Part model, mm, in its own coordinate system. Face numbers are marked on the shaded views. Round coordinates to 2 decimals unless told otherwise and drop trailing zeros. Loops run counter-clockwise (first coordinate to the right, second up) from the corner with the lowest first, then second, coordinate; pieces in that order, holes last.
1) Band-saw the part on A-A, the plane x = -49. Write the cut outline in (y, z), then the cut area to 3 significant figures.
2) Drop flat-ended pins along their axis: P1, Ø0.5, axis at x = 59, y = 0.5, coming from the +Z side; P2, Ø5, axis at x = 72.5, z = 68, coming from the -Y side; P3, Ø1, axis at y = 10.5, z = -46.5, coming from the -X side; P4, Ø2.5, axis at x = -72.5, z = -68, coming from the +Y side. Give the stop position or say it passes through.
3) Probe line 1 (X direction, y = 5.3, z = -68); line 2 (Z direction, x = 2.5, y = 6.25); line 3 (Z direction, x = 72.5, y = 4.6). List the from-to ranges inside material, lowest first.
4) Band-saw the part on B-B, the plane z = 12. Write the cut outline in (x, y).
5) Mould opens along X. For the marked faces 1, 2 and 3 say: +X half, -X half, draft (parallel to the pull), parting line (faces both ways), or undercut.
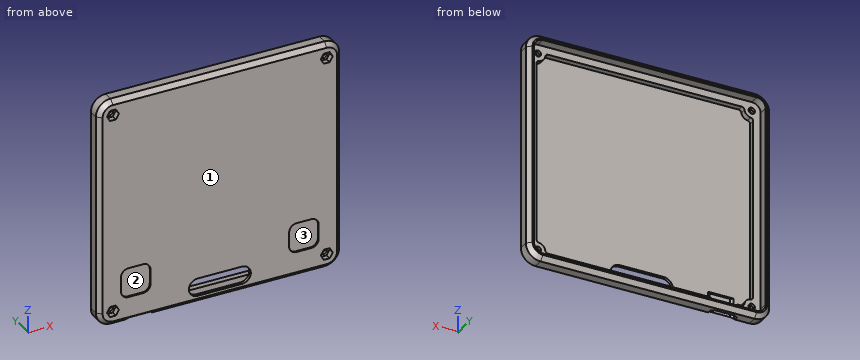
from build123d import *

# Parameters (mm, degrees)
BOSS_EXTRUDE2_DEPTH      = 2
BOSS_EXTRUDE3_DEPTH      = 4
BOSS_EXTRUDE3_DEPTH_BACK = 2
SKETCH3_R                = 2.15
BOSS_EXTRUDE4_DEPTH      = 6.38
CUT_EXTRUDE1_DEPTH       = 15
FILLET1_R                = 2
CUT_EXTRUDE3_DEPTH       = 115.008747033
CUT_EXTRUDE3_DEPTH_BACK  = 115.008747033
SKETCH11_R               = 2.15
CUT_EXTRUDE2_DEPTH       = 4
CHAMFER1_SIZE            = 3
SKETCH13_W               = 18
SKETCH13_H               = 5
CUT_EXTRUDE5_DEPTH       = 1
CUT_EXTRUDE6_DEPTH       = 1
CUT_EXTRUDE7_DEPTH       = 2


with BuildPart() as part:
    # Sketch2 → Boss-Extrude2 (new body)
    with BuildSketch(Plane(origin=(0, 0, 0), x_dir=(1, 0, 0), z_dir=(0, 1, 0))):
        with BuildLine():
            Line((-72.5, 74), (72.5, 74))
            ThreePointArc((72.5, 74), (76.742640687, 72.242640687), (78.5, 68))
            Line((78.5, 68), (78.5, -68))
            ThreePointArc((78.5, -68), (76.742640687, -72.242640687), (72.5, -74))
            Line((72.5, -74), (-72.5, -74))
            ThreePointArc((-72.5, -74), (-76.742640687, -72.242640687), (-78.5, -68))
            Line((-78.5, -68), (-78.5, 68))
            ThreePointArc((-78.5, 68), (-76.742640687, 72.242640687), (-72.5, 74))
        make_face()
    extrude(amount=BOSS_EXTRUDE2_DEPTH)

    # Sketch3 → Boss-Extrude3 (add, two sides: drawn at the far end of the back side and taken through both)
    with BuildSketch(Plane(origin=(0, 2, 0), x_dir=(1, 0, 0), z_dir=(0, 1, 0)).offset(-BOSS_EXTRUDE3_DEPTH_BACK)):
        with BuildLine():
            Line((-82.5, 68), (-82.5, -68))
            ThreePointArc((-82.5, -68), (-79.571067812, -75.071067812), (-72.5, -78))
            Line((-72.5, -78), (72.5, -78))
            ThreePointArc((72.5, -78), (79.571067812, -75.071067812), (82.5, -68))
            Line((82.5, -68), (82.5, 68))
            ThreePointArc((82.5, 68), (79.571067812, 75.071067812), (72.5, 78))
            Line((72.5, 78), (-72.5, 78))
            ThreePointArc((-72.5, 78), (-79.571067812, 75.071067812), (-82.5, 68))
        make_face()
        with Locations(Location((-72.5, -68, 0), (0, 0, 270))):
            Circle(SKETCH3_R, mode=Mode.SUBTRACT)
        with Locations(Location((72.5, -68, 0), (0, 0, 270))):
            Circle(SKETCH3_R, mode=Mode.SUBTRACT)
        with Locations(Location((72.5, 68, 0), (0, 0, 270))):
            Circle(SKETCH3_R, mode=Mode.SUBTRACT)
        with Locations(Location((-72.5, 68, 0), (0, 0, 270))):
            Circle(SKETCH3_R, mode=Mode.SUBTRACT)
        with BuildLine():
            Line((-73.5, 63), (-73.5, -63))
            Line((-73.5, -63), (-72.5, -63))
            ThreePointArc((-72.5, -63), (-68.964466094, -64.464466094), (-67.5, -68))
            Line((-67.5, -68), (-67.5, -69))
            Line((-67.5, -69), (67.5, -69))
            Line((67.5, -69), (67.5, -68))
            ThreePointArc((67.5, -68), (68.964466094, -64.464466094), (72.5, -63))
            Line((72.5, -63), (73.5, -63))
            Line((73.5, -63), (73.5, 63))
            Line((73.5, 63), (72.5, 63))
            ThreePointArc((72.5, 63), (68.964466094, 64.464466094), (67.5, 68))
            Line((67.5, 68), (67.5, 69))
            Line((67.5, 69), (-67.5, 69))
            Line((-67.5, 69), (-67.5, 68))
            ThreePointArc((-67.5, 68), (-68.964466094, 64.464466094), (-72.5, 63))
            Line((-72.5, 63), (-73.5, 63))
        make_face(mode=Mode.SUBTRACT)
    extrude(amount=BOSS_EXTRUDE3_DEPTH + BOSS_EXTRUDE3_DEPTH_BACK)

    # Sketch8 → Boss-Extrude4 (add)
    with BuildSketch(Plane(origin=(0, 6, 0), x_dir=(1, 0, 0), z_dir=(0, 1, 0))):
        with BuildLine():
            ThreePointArc((82.5, 68), (79.571067812, 75.071067812), (72.5, 78))
            Line((72.5, 78), (-72.5, 78))
            ThreePointArc((-72.5, 78), (-79.571067812, 75.071067812), (-82.5, 68))
            Line((-82.5, 68), (-82.5, -68))
            ThreePointArc((-82.5, -68), (-79.571067812, -75.071067812), (-72.5, -78))
            Line((-72.5, -78), (72.5, -78))
            ThreePointArc((72.5, -78), (79.571067812, -75.071067812), (82.5, -68))
            Line((82.5, -68), (82.5, 68))
        make_face()
        with BuildLine():
            ThreePointArc((72.5, -74), (76.742640687, -72.242640687), (78.5, -68))
            Line((78.5, -68), (78.5, 68))
            ThreePointArc((78.5, 68), (76.742640687, 72.242640687), (72.5, 74))
            Line((72.5, 74), (-72.5, 74))
            ThreePointArc((-72.5, 74), (-76.742640687, 72.242640687), (-78.5, 68))
            Line((-78.5, 68), (-78.5, -68))
            ThreePointArc((-78.5, -68), (-76.742640687, -72.242640687), (-72.5, -74))
            Line((-72.5, -74), (72.5, -74))
        make_face(mode=Mode.SUBTRACT)
    extrude(amount=BOSS_EXTRUDE4_DEPTH)

    # Sketch9 → Cut-Extrude1 (cut)
    with BuildSketch(Plane(origin=(0, 0, -78), x_dir=(-1, 0, 0), z_dir=(0, 0, -1))):
        Polygon((60.62, 7.11), (46.62, 7.11), (44.62, 5.51), (44.62, 2.19), (46.62, 0.59), (60.62, 0.59), (62.62, 2.19), (62.62, 5.51), align=None)
    extrude(amount=-CUT_EXTRUDE1_DEPTH, mode=Mode.SUBTRACT)

    # Fillet1
    fillet1_edges = [part.edges().sort_by_distance(p)[0] for p in [
        (-67.5, 4, -69),
        (-73.5, 4, -63),
        (-73.5, 4, 63),
        (-67.5, 4, 69),
        (73.5, 4, 63),
        (67.5, 4, 69),
        (67.5, 4, -69),
        (73.5, 4, -63),
    ]]
    fillet(fillet1_edges, radius=FILLET1_R)

    # Sketch11 → Cut-Extrude3 (cut, two sides: drawn at the far end of the back side and taken through both)
    with BuildSketch(Plane(origin=(0, 2, 0), x_dir=(1, 0, 0), z_dir=(0, 1, 0)).offset(-CUT_EXTRUDE3_DEPTH_BACK)):
        with Locations(Location((-72.5, -68, 0), (0, 0, 270))):
            Circle(SKETCH11_R)
        with Locations(Location((72.5, -68, 0), (0, 0, 270))):
            Circle(SKETCH11_R)
        with Locations(Location((72.5, 68, 0), (0, 0, 270))):
            Circle(SKETCH11_R)
        with Locations(Location((-72.5, 68, 0), (0, 0, 270))):
            Circle(SKETCH11_R)
    extrude(amount=CUT_EXTRUDE3_DEPTH + CUT_EXTRUDE3_DEPTH_BACK, mode=Mode.SUBTRACT)

    # Sketch10 → Cut-Extrude2 (cut)
    with BuildSketch(Plane.XZ):
        Polygon((-74.520725942, 64.5), (-70.479274058, 64.5), (-68.458548116, 68), (-70.479274058, 71.5), (-74.520725942, 71.5), (-76.541451884, 68), align=None)
        Polygon((76.541451884, 68), (74.520725942, 64.5), (70.479274058, 64.5), (68.458548116, 68), (70.479274058, 71.5), (74.520725942, 71.5), align=None)
        Polygon((-70.479274058, -64.5), (-68.458548116, -68), (-70.479274058, -71.5), (-74.520725942, -71.5), (-76.541451884, -68), (-74.520725942, -64.5), align=None)
        Polygon((76.541451884, -68), (74.520725942, -64.5), (70.479274058, -64.5), (68.458548116, -68), (70.479274058, -71.5), (74.520725942, -71.5), align=None)
    extrude(amount=-CUT_EXTRUDE2_DEPTH, mode=Mode.SUBTRACT)

    # Chamfer1
    # the kernel refuses this chamfer: 3 mm, written as the material it takes off along each edge
    with BuildSketch(Plane(origin=(-72.5, 12.38, 68), x_dir=(-1, 0, 0), z_dir=(0, 0, -1))) as chamfer1_piece_1:
        Polygon((10 - CHAMFER1_SIZE, 0), (10, -CHAMFER1_SIZE), (10, 0), align=None)
    revolve(axis=Axis((-72.5, 12.38, 68), (0, 1, 0)), revolution_arc=90, mode=Mode.SUBTRACT)
    with BuildSketch(Plane(origin=(-72.5, 12.38, 78), x_dir=(0, 0.02749587661058619, -0.9996219169112968), z_dir=(1, 0, 0)), Plane(origin=(72.5, 0, -78), x_dir=(0, 0.9996219169112968, -0.027495876610586778), z_dir=(-1, 0, 0))) as chamfer1_piece_2:
        Polygon((CHAMFER1_SIZE * 0.999621916911, -CHAMFER1_SIZE * 0.0274958766106), (-CHAMFER1_SIZE * 0.0274958766106, -CHAMFER1_SIZE * 0.999621916911), (0, 0), align=None)
    extrude(amount=145, mode=Mode.SUBTRACT)
    with BuildSketch(Plane(origin=(72.5, 12.38, 68), x_dir=(0, 0, 1), z_dir=(-1, 0, 0))) as chamfer1_piece_3:
        Polygon((10 - CHAMFER1_SIZE, 0), (10, -CHAMFER1_SIZE), (10, 0), align=None)
    revolve(axis=Axis((72.5, 12.38, 68), (0, 1, 0)), revolution_arc=90, mode=Mode.SUBTRACT)
    with BuildSketch(Plane(origin=(82.5, 12.38, 68), x_dir=(-0.9996219169112968, 0.02749587661058619, 0), z_dir=(0, 0, -1)), Plane(origin=(-82.5, 12.38, -68), x_dir=(0.9996219169112968, 0.02749587661058619, 0), z_dir=(0, 0, 1))) as chamfer1_piece_4:
        Polygon((CHAMFER1_SIZE * 0.999621916911, -CHAMFER1_SIZE * 0.0274958766106), (-CHAMFER1_SIZE * 0.0274958766106, -CHAMFER1_SIZE * 0.999621916911), (0, 0), align=None)
    extrude(amount=136, mode=Mode.SUBTRACT)
    with BuildSketch(Plane(origin=(72.5, 12.38, -68), x_dir=(1, 0, 0), z_dir=(0, 0, 1))) as chamfer1_piece_5:
        Polygon((10 - CHAMFER1_SIZE, 0), (10, -CHAMFER1_SIZE), (10, 0), align=None)
    revolve(axis=Axis((72.5, 12.38, -68), (0, 1, 0)), revolution_arc=90, mode=Mode.SUBTRACT)
    with BuildSketch(Plane(origin=(72.5, 12.38, -78), x_dir=(0, -0.9996219169112968, -0.02749587661058678), z_dir=(-1, 0, 0)), Plane(origin=(-72.5, 0, 78), x_dir=(0, -0.02749587661058636, -0.9996219169112968), z_dir=(1, 0, 0))) as chamfer1_piece_6:
        Polygon((CHAMFER1_SIZE * 0.999621916911, CHAMFER1_SIZE * 0.0274958766106), (-CHAMFER1_SIZE * 0.0274958766106, CHAMFER1_SIZE * 0.999621916911), (0, 0), align=None)
    extrude(amount=145, mode=Mode.SUBTRACT)
    with BuildSketch(Plane(origin=(-72.5, 12.38, -68), x_dir=(0, 0, -1), z_dir=(1, 0, 0))) as chamfer1_piece_7:
        Polygon((10 - CHAMFER1_SIZE, 0), (10, -CHAMFER1_SIZE), (10, 0), align=None)
    revolve(axis=Axis((-72.5, 12.38, -68), (0, 1, 0)), revolution_arc=90, mode=Mode.SUBTRACT)
    with BuildSketch(Plane(origin=(-72.5, 0, -68), x_dir=(0, 0, -1), z_dir=(1, 0, 0))) as chamfer1_piece_8:
        Polygon((10 - CHAMFER1_SIZE, 0), (10, CHAMFER1_SIZE), (10, 0), align=None)
    revolve(axis=Axis((-72.5, 0, -68), (0, 1, 0)), revolution_arc=90, mode=Mode.SUBTRACT)
    with BuildSketch(Plane(origin=(-82.5, 0, -68), x_dir=(0.9996219169112968, -0.02749587661058636, 0), z_dir=(0, 0, 1)), Plane(origin=(82.5, 0, 68), x_dir=(-0.9996219169112968, -0.02749587661058636, 0), z_dir=(0, 0, -1))) as chamfer1_piece_9:
        Polygon((CHAMFER1_SIZE * 0.999621916911, CHAMFER1_SIZE * 0.0274958766106), (-CHAMFER1_SIZE * 0.0274958766106, CHAMFER1_SIZE * 0.999621916911), (0, 0), align=None)
    extrude(amount=136, mode=Mode.SUBTRACT)
    with BuildSketch(Plane(origin=(-72.5, 0, 68), x_dir=(-1, 0, 0), z_dir=(0, 0, -1))) as chamfer1_piece_10:
        Polygon((10 - CHAMFER1_SIZE, 0), (10, CHAMFER1_SIZE), (10, 0), align=None)
    revolve(axis=Axis((-72.5, 0, 68), (0, 1, 0)), revolution_arc=90, mode=Mode.SUBTRACT)
    with BuildSketch(Plane(origin=(72.5, 0, 68), x_dir=(0, 0, 1), z_dir=(-1, 0, 0))) as chamfer1_piece_11:
        Polygon((10 - CHAMFER1_SIZE, 0), (10, CHAMFER1_SIZE), (10, 0), align=None)
    revolve(axis=Axis((72.5, 0, 68), (0, 1, 0)), revolution_arc=90, mode=Mode.SUBTRACT)
    with BuildSketch(Plane(origin=(72.5, 0, -68), x_dir=(1, 0, 0), z_dir=(0, 0, 1))) as chamfer1_piece_12:
        Polygon((10, CHAMFER1_SIZE), (10 - CHAMFER1_SIZE, 0), (10, 0), align=None)
    revolve(axis=Axis((72.5, 0, -68), (0, 1, 0)), revolution_arc=90, mode=Mode.SUBTRACT)

    # Sketch13 → Cut-Extrude5 (cut)
    with BuildSketch(Plane(origin=(0, 6, 0), x_dir=(1, 0, 0), z_dir=(0, 1, 0))):
        with Locations((-53.62, 71.5)):
            Rectangle(SKETCH13_W, SKETCH13_H)
    extrude(amount=-CUT_EXTRUDE5_DEPTH, mode=Mode.SUBTRACT)

    # Sketch14 → Cut-Extrude6 (cut)
    with BuildSketch(Plane.XZ):
        with BuildLine():
            Line((-62, -41), (-52, -41))
            ThreePointArc((-52, -41), (-48.464466094, -42.464466094), (-47, -46))
            Line((-47, -46), (-47, -56))
            ThreePointArc((-47, -56), (-48.464466094, -59.535533906), (-52, -61))
            Line((-52, -61), (-62, -61))
            ThreePointArc((-62, -61), (-65.535533906, -59.535533906), (-67, -56))
            Line((-67, -56), (-67, -46))
            ThreePointArc((-67, -46), (-65.535533906, -42.464466094), (-62, -41))
        make_face()
        with BuildLine():
            Line((62, -61), (52, -61))
            ThreePointArc((52, -61), (48.464466094, -59.535533906), (47, -56))
            Line((47, -56), (47, -46))
            ThreePointArc((47, -46), (48.464466094, -42.464466094), (52, -41))
            Line((52, -41), (62, -41))
            ThreePointArc((62, -41), (65.535533906, -42.464466094), (67, -46))
            Line((67, -46), (67, -56))
            ThreePointArc((67, -56), (65.535533906, -59.535533906), (62, -61))
        make_face()
    extrude(amount=-CUT_EXTRUDE6_DEPTH, mode=Mode.SUBTRACT)

    # Sketch15 → Cut-Extrude7 (cut)
    with BuildSketch(Plane.XZ):
        with BuildLine():
            Line((-15, -61), (15, -61))
            ThreePointArc((15, -61), (21, -67), (15, -73))
            Line((15, -73), (-15, -73))
            ThreePointArc((-15, -73), (-21, -67), (-15, -61))
        make_face()
    extrude(amount=-CUT_EXTRUDE7_DEPTH, mode=Mode.SUBTRACT)


solid = part.part
Reported:
1. outline: (0, -75) - (0.59, -75.59) - (0.59, -63) - (2, -63) - (2, 69) - (6, 69) - (6, 74) - (12.38, 74) - (12.38, 75) - (9.38, 78) - (3, 78) - (0, 75) - (0, -42) - (1, -42) - (1, -60) - (0, -60) - close; (7.11, -78) - (9.38, -78) - (12.38, -75) - (12.38, -74) - (7.11, -74) - close
1. area: 340 mm2
2. P1: stops at z = 75.75
2. P2: stops at y = 4
2. P3: stops at x = -81.88
2. P4: passes through
3. line 1: x = -82.5 to -74.65, -70.35 to -67.3, 67.3 to 70.35, 74.65 to 82.5
3. line 2: z = -78 to -74, 74 to 78
3. line 3: z = -78 to -70.15, -65.85 to -62.8, 62.8 to 65.85, 70.15 to 78
4. outline: (-82.5, 3) - (-79.5, 0) - (79.5, 0) - (82.5, 3) - (82.5, 9.38) - (79.5, 12.38) - (78.5, 12.38) - (78.5, 6) - (73.5, 6) - (73.5, 2) - (-73.5, 2) - (-73.5, 6) - (-78.5, 6) - (-78.5, 12.38) - (-79.5, 12.38) - (-82.5, 9.38) - close
5. face 1: draft
5. face 2: undercut
5. face 3: undercut
